```python
from build123d import *

# Parameters (mm, degrees)
F0_R      = 13.423157
F1_DEPTH  = 37.846
F2_R      = 12.877415
F1_FACE_R = 0.545742
F3_DEPTH  = 6.604


with BuildPart() as f1:
    # F0 (on Top) → F1 (new body)
    with BuildSketch(Plane.XY):
        Circle(F0_R)
    extrude(amount=F1_DEPTH)

    # F2
    f2_edges = [f1.edges().sort_by_distance(p)[0] for p in [
        (-13.423157, 0, 37.846),
    ]]
    fillet(f2_edges, radius=F2_R)

    # F1_face (on face) → F3 (join)
    with BuildSketch(Plane.XY.offset(37.846)):
        Circle(F1_FACE_R)
    extrude(amount=F3_DEPTH)


solid = f1.part
```
Verification items for the finished model (mm, model axes). A direction names the side the tool comes from. Round coordinates to 2 decimals unless told otherwise and drop trailing zeros. Order: outer loops, then holes, each group sorted by start corner. A loop starts at its lowest first (then second) coordinate and runs counter-clockwise, first axis right, second up.
1) Cross-section at B-B, the plane z = 18.5. Record the cut outline in (x, y), plus the area to 3 significant figures.
Geometry says:
outline: circle Ø26.85 at (0, 0)
area: 566 mm2
2) Tool access check on faces 1 (the cylindrical face through (-0.433, -0.332, 41.102)), 2 (the flat face through (0, 0, 44.45)). Record the directions out of +Z, -Z, +X, -X, +Y, -Y that give a thin tool (end or side, any length) a straight path to the whole face; none if there is none.
Geometry says:
face 1: +Z
face 2: +Z, +X, -X, +Y, -Y
3) Cross-section at A-A, the plane z = 38.5. Record the cut outline in (x, y).
Geometry says:
outline: circle Ø1.09 at (0, 0)
4) Depth check by flat-ended pin: pin 1 (12 mm diameter, centred on x = -9.5, y = 8.5, fed in from -Z); pin 2 (2 mm diameter, centred on y = -8.5, z = 8.5, fed in from +X); pin 3 (8 mm diameter, centred on y = 10, z = 16, fed in from -X); pin 4 (1 mm diameter, centred on x = -8.5, y = -4, fed in from +Z). Enter the tip coordinate at first touch or a pass-through.
Geometry says:
pin 1: stops at z = 0
pin 2: stops at x = 11.13
pin 3: stops at x = -12.01
pin 4: stops at z = 34.77
5) Material ranges on line 1 (Y direction, x = -0.5, z = 18.5); line 2 (Y direction, x = -11, z = 3); line 3 (Z direction, x = 10.5, y = 0.25), recorded low to high.
Geometry says:
line 1: y = -13.41 to 13.41
line 2: y = -7.69 to 7.69
line 3: z = 0 to 33.13
